Source: CAD feature listing. Evaluate the final solid. Frame: model axes, mm. Coordinates: 2 decimals unless noted, no trailing zeros. Write each loop counter-clockwise with the first axis right and the second up, starting at its lowest first coordinate (ties: lowest second). Pieces come first, ordered by that corner, then holes. Notation, with made-up numbers: M 62,68 L 106,68 A32 cw 106,98 Z; hole C 3,61.25 d6. An arc over 180 degrees is marked long. One line per item, written item: value. Start each with the question number.
Item 1: Cut plane C-C, the plane z = 1. Output: boundary loops of the cut face in (x, y), then the cut area to 3 significant figures.
Item 2: Cut plane A-A, the plane y = -11. Output: boundary loops of the cut face in (x, z), then the cut area to 3 significant figures.
Item 3: Cut plane B-B, the plane x = 0.35. Output: boundary loops of the cut face in (y, z) (3 decimals).
Item 4: Pin query (flat end, axial travel): P1, Ø0.8, axis at x = 0, y = -6.5, coming from the +Z side. Return the tip coordinate at first contact, or that it passes through.
Item 5: Cut plane D-D, the plane y = 1.5. Output: boundary loops of the cut face in (x, z).
Item 6: Ray query, L1, parallel to Z at x = 0.6, y = 0 (3 decimals); L2, parallel to Z at x = 0.3, y = 1; L3, parallel to Y at x = -0.55, z = 2.5. Return the intervals inside material, ascending. Write a range as from..to.
```python
from build123d import *

# Parameters (mm, degrees)
F0_R     = 3.175
F1_DEPTH = 1.25


with BuildPart() as f1:
    # F0 (on Right) → F1 (new body, symmetric)
    with BuildSketch(Plane.YZ):
        with BuildLine():
            Line((-24, 10), (-24, 0))
            ThreePointArc((-24, 0), (-17.054114, -17.493789), (0, -25.458409))
            Line((0, -25.458409), (60, -29))
            Line((60, -29), (61, -18))
            Line((61, -18), (23, -12))
            Line((23, -12), (19, -9))
            Line((19, -9), (15, 13))
            Line((15, 13), (8, 13))
            Line((8, 13), (6, 10))
            Line((6, 10), (-24, 10))
        make_face()
        with BuildLine():
            ThreePointArc((-19.226374, 3.362237), (-16.931961, 5.016223), (-15.277975, 2.721811))
            ThreePointArc((-15.277975, 2.721811), (-10.850381, -11.679078), (3.279705, -16.906872))
            ThreePointArc((3.279705, -16.906872), (5.477806, -18.686859), (3.697819, -20.88496))
            ThreePointArc((3.697819, -20.88496), (-13.756994, -14.427096), (-19.226374, 3.362237))
        make_face(mode=Mode.SUBTRACT)
        Circle(F0_R, mode=Mode.SUBTRACT)
    extrude(amount=F1_DEPTH, both=True)


solid = f1.part
```
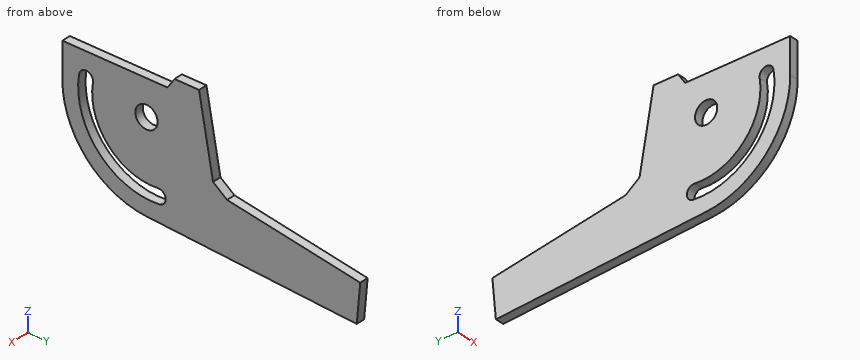
From the geometry:
1. outline: M -1.25,-24 L 1.25,-24 L 1.25,-19.47 L -1.25,-19.47 Z; M -1.25,-15.47 L 1.25,-15.47 L 1.25,-3.01 L -1.25,-3.01 Z; M -1.25,3.01 L 1.25,3.01 L 1.25,17.18 L -1.25,17.18 Z
1. area: 77.9 mm²
2. outline: M -1.25,-22.23 L 1.25,-22.23 L 1.25,-16.87 L -1.25,-16.87 Z; M -1.25,-11.52 L 1.25,-11.52 L 1.25,10 L -1.25,10 Z
2. area: 67.2 mm²
3. outline: M -24,0 A25.503 ccw 0,-25.458 L 60,-29 L 61,-18 L 23,-12 L 19,-9 L 15,13 L 8,13 L 6,10 L -24,10 Z; hole M -19.226,3.362 A21 ccw 3.698,-20.885 A2 ccw 3.28,-16.907 A17 cw -15.278,2.722 A2 ccw Z; hole C 0,0 d6.35
4. P1: stops at z = 10
5. outline: M -1.25,-25.55 L 1.25,-25.55 L 1.25,-21 L -1.25,-21 Z; M -1.25,-17 L 1.25,-17 L 1.25,-2.8 L -1.25,-2.8 Z; M -1.25,2.8 L 1.25,2.8 L 1.25,10 L -1.25,10 Z
6. L1: z = -25.458..-20.946, -16.933..-3.175, 3.175..10
6. L2: z = -25.52..-20.99, -16.99..-3.01, 3.01..10
6. L3: y = -24..-19.35, -15.31..-1.96, 1.96..16.91
